Geometry check sheet. Reference: the model listing, model coordinates, mm. Round coordinates to 2 decimals unless told otherwise and drop trailing zeros. Order: outer loops, then holes, each group sorted by start corner. A loop starts at its lowest first (then second) coordinate and runs counter-clockwise, first axis right, second up.
```python
from build123d import *

# Parameters (mm, degrees)
SKETCH1_R           = 6.715
BOSS_EXTRUDE1_DEPTH = 5
FILLET1_R           = 1
CUT_EXTRUDE1_REACH  = 12.732
SKETCH2_R           = 1


with BuildPart() as part:
    # Sketch1 → Boss-Extrude1 (new body)
    with BuildSketch(Plane(origin=(0, 0, 0), x_dir=(1, 0, 0), z_dir=(0, 1, 0))):
        with Locations(Location((0, 0, 0), (0, 0, 270))):
            Circle(SKETCH1_R)
    extrude(amount=BOSS_EXTRUDE1_DEPTH)

    # Fillet1
    fillet1_edges = [part.edges().sort_by_distance(p)[0] for p in [
        (0, 0, -6.715),
        (0, 5, -6.715),
    ]]
    fillet(fillet1_edges, radius=FILLET1_R)

    # Sketch2 → Cut-Extrude1 (cut, up to next)
    with BuildSketch(Plane(origin=(0, 5, 0), x_dir=(1, 0, 0), z_dir=(0, 1, 0)), mode=Mode.PRIVATE) as cut_extrude1_sk1:
        with Locations(Location((0, 0, 0), (0, 0, 270))):
            Circle(SKETCH2_R)
    cut_extrude1_tool1 = extrude(cut_extrude1_sk1.sketch, amount=-CUT_EXTRUDE1_REACH, mode=Mode.PRIVATE) & part.part
    add(cut_extrude1_tool1.solids().sort_by_distance((0, 5, 0))[0], mode=Mode.SUBTRACT)


solid = part.part
```
(1) Sectioned sample at A-A, the plane z = 0. Record the cut outline in (x, y) (3 decimals).
Returned:
outline: (-6.715, 1) arc R1 ccw to (-5.715, 0) - (-1, 0) - (-1, 5) - (-5.715, 5) arc R1 ccw to (-6.715, 4) - close; (1, 0) - (5.715, 0) arc R1 ccw to (6.715, 1) - (6.715, 4) arc R1 ccw to (5.715, 5) - (1, 5) - close
(2) Sectioned sample at B-B, the plane x = 0. Record the cut outline in (y, z) (3 decimals), and give its area (3 significant figures).
Returned:
outline: (0, -5.715) arc R1 ccw to (1, -6.715) - (4, -6.715) arc R1 ccw to (5, -5.715) - (5, -1) - (0, -1) - close; (0, 1) - (5, 1) - (5, 5.715) arc R1 ccw to (4, 6.715) - (1, 6.715) arc R1 ccw to (0, 5.715) - close
area: 56.3 mm2
(3) Draft check along X on faces 1 (the cylindrical face through (-2.572, 2.479, 6.203)), 2 (the cylindrical face through (-1, 3, 0)), 3 (the flat face through (-1.2, 5, -0.1)). Enter one of: released by +X, released by -X, zero draft, split by the parting line, or undercut.
Returned:
face 1: split by the parting line
face 2: undercut
face 3: zero draft
(4) Sectioned sample at D-D, the plane y = 4.75. Record the cut outline in (x, z), and give its area (3 significant figures).
Returned:
outline: circle Ø12.75 at (0, 0); hole circle Ø2 at (0, 0)
area: 125 mm2
(5) Sectioned sample at C-C, the plane y = 3.3. Record the cut outline in (x, z) (3 decimals), and give its area (3 significant figures).
Returned:
outline: circle Ø13.43 at (0, 0); hole circle Ø2 at (0, 0)
area: 139 mm2
(6) Material ranges on line 1 (X direction, y = 3.85, z = 0) (3 decimals); line 2 (Z direction, x = 0.25, y = 1.85); line 3 (Z direction, x = 0.75, y = 4.5), recorded low to high.
Returned:
line 1: x = -6.715 to -1, 1 to 6.715
line 2: z = -6.71 to -0.97, 0.97 to 6.71
line 3: z = -6.54 to -0.66, 0.66 to 6.54
(7) Depth check by flat-ended pin: P1, Ø1, axis at x = 3, y = 3.5, coming from the -Z side; P2, Ø1.5, axis at y = 1.5, z = -1.5, coming from the +X side; P3, Ø1, axis at y = 1.5, z = -4.5, coming from the -X side. Enter the tip coordinate at first touch or a pass-through.
Returned:
P1: stops at z = -6.23
P2: stops at x = 6.67
P3: stops at x = -5.39
